For this review, use the dimensioned drawing (mm, ordinates from the lowest corner) and the shaded views. A direction names the side the tool comes from. Round coordinates to 2 decimals unless told otherwise and drop trailing zeros. Order: outer loops, then holes, each group sorted by start corner. A loop starts at its lowest first (then second) coordinate and runs counter-clockwise, first axis right, second up. Notation, with made-up numbers: (15.5, 16.5) -> (65.5, 16.5) arc R21 cw to (65.5, 47.5) -> close; hole circle Ø7 at (-10, -24.5). An arc over 180 degrees is marked (long way). Answer in a Markdown table with one row per item.
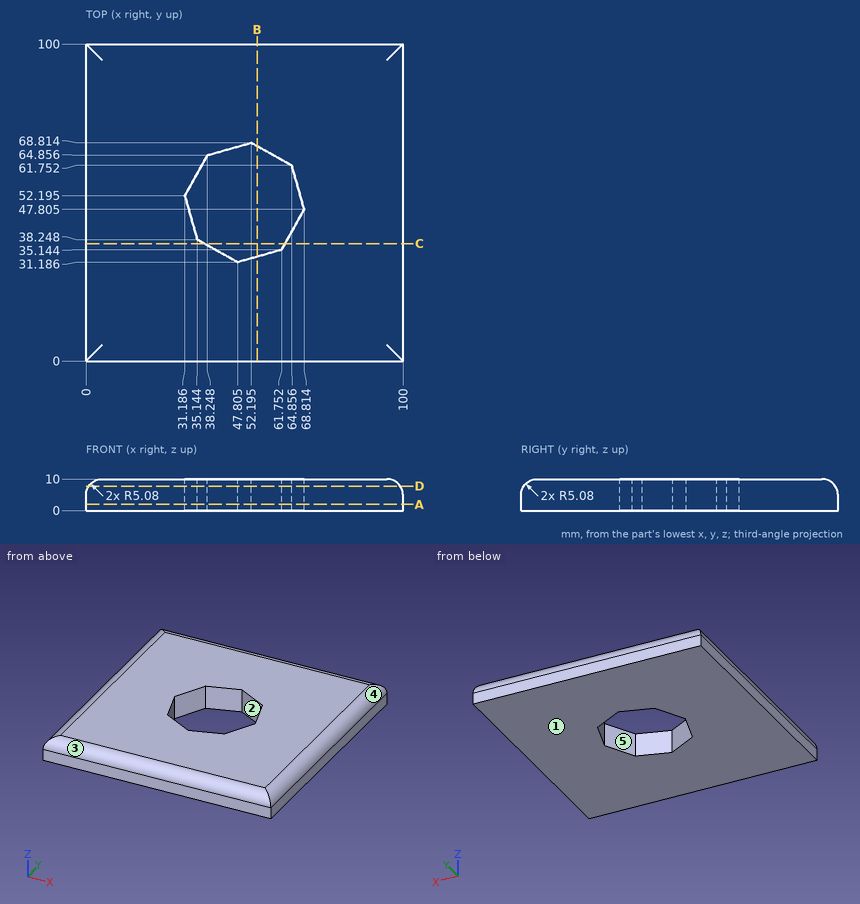
Q1. Clearance check with a flat-ended pin moving along its axis: pin 1 Ø3 at (y, z) = (35.5, 7) entering from -X. State where the tip first meets the part, or that it passes through.
Answer key:
| item | result |
|---|---|
| pin 1 | stops at x = 0.03 |
Q2. Tool access review of the marked faces 4 and 5: name each direction out of +Z, -Z, +X, -X, +Y, -Y from which nothing blocks a thin tool from reaching the whole face with its end or side.
Answer key:
| item | result |
|---|---|
| face 4 | +Z, +X, +Y, -Y |
| face 5 | +Z, -Z |
Q3. Take a section at C-C, the plane y = 37. Write out the cut boundary in (x, z), then the cut area to 3 significant figures.
Answer key:
| item | result |
|---|---|
| outline | (0, 0) -> (37.38, 0) -> (37.38, 10) -> (5.08, 10) arc R5.08 ccw to (0, 4.92) -> close; (62.79, 0) -> (100, 0) -> (100, 4.92) arc R5.08 ccw to (94.92, 10) -> (62.79, 10) -> close |
| area | 735 mm^2 |
Q4. Take a section at D-D, the plane z = 7.75. Write out the cut boundary in (x, y) (1 decimal), then the cut area to 3 significant figures.
Answer key:
| item | result |
|---|---|
| outline | (0.9, 0.9) -> (99.1, 0.9) -> (99.1, 99.1) -> (0.9, 99.1) -> close; hole (31.2, 52.2) -> (35.1, 38.2) -> (47.8, 31.2) -> (61.8, 35.1) -> (68.8, 47.8) -> (64.9, 61.8) -> (52.2, 68.8) -> (38.2, 64.9) -> close |
| area | 8,640 mm^2 |
Q5. Take a section at A-A, the plane z = 2. Write out the cut boundary in (x, y) (1 decimal).
Answer key:
| item | result |
|---|---|
| outline | (0, 0) -> (100, 0) -> (100, 100) -> (0, 100) -> close; hole (31.2, 52.2) -> (35.1, 38.2) -> (47.8, 31.2) -> (61.8, 35.1) -> (68.8, 47.8) -> (64.9, 61.8) -> (52.2, 68.8) -> (38.2, 64.9) -> close |
Q6. To check wall thickness, follow probe 1 along X at (y, z) = (49, 8.5) (1 decimal); probe 2 along X at (y, z) = (36.5, 9.25) (1 decimal); probe 3 along Y at (x, z) = (43.5, 4.5) (1 decimal). State the ranges of each line that lie inside material, in increasing order.
Answer key:
| item | result |
|---|---|
| probe 1 | x = 1.5 to 32.1, 68.5 to 98.5 |
| probe 2 | x = 2.4 to 38.3, 62.5 to 97.6 |
| probe 3 | y = 0 to 33.6, 66.3 to 100 |
Q7. The part is to be moulded in two halves that separate along Y. For the marked faces 1, 2 and 3, say which applies: +Y half, -Y half, draft (parallel to the pull), parting line (faces both ways), or undercut.
Answer key:
| item | result |
|---|---|
| face 1 | draft |
| face 2 | undercut |
| face 3 | -Y half |
Q8. Take a section at B-B, the plane x = 54. Write out the cut boundary in (y, z) (1 decimal), then the cut area to 3 significant figures.
Answer key:
| item | result |
|---|---|
| outline | (0, 0) -> (32.9, 0) -> (32.9, 10) -> (5.1, 10) arc R5.1 ccw to (0, 4.9) -> close; (67.8, 0) -> (100, 0) -> (100, 4.9) arc R5.1 ccw to (94.9, 10) -> (67.8, 10) -> close |
| area | 640 mm^2 |
